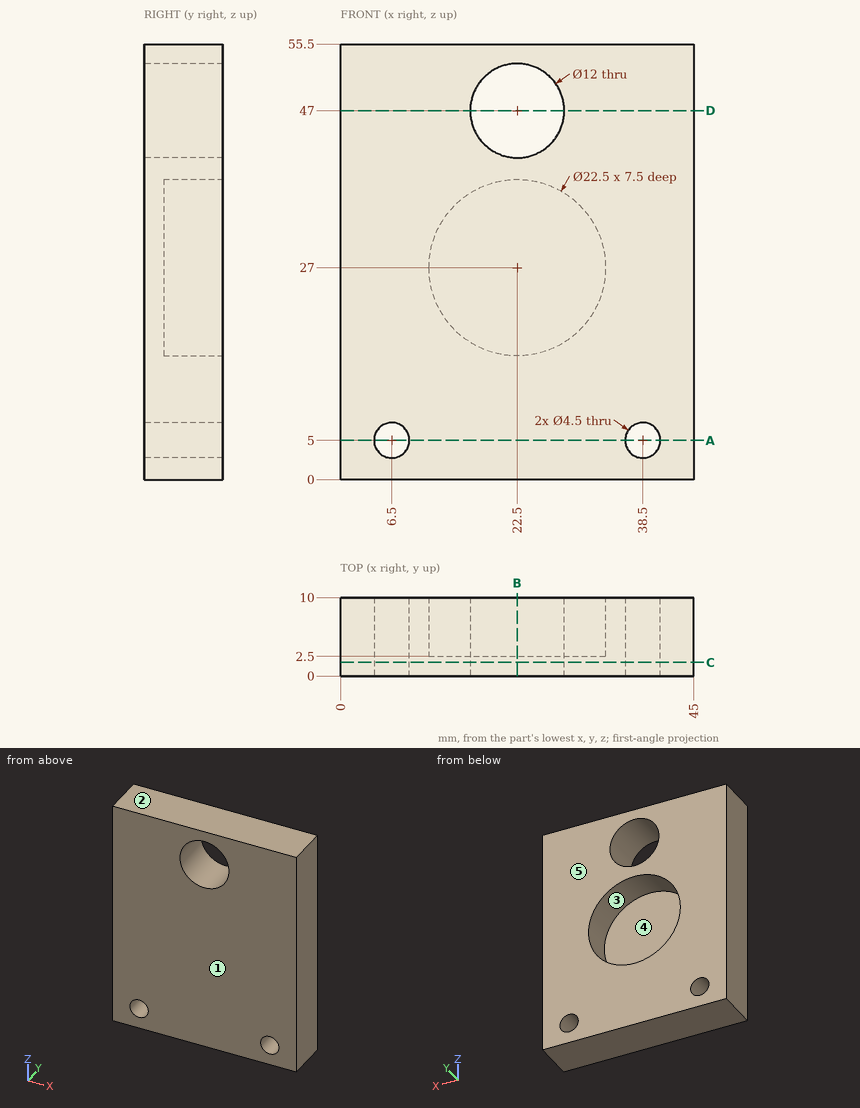
The drawing under review shows one solid part. Ordinate dimensions are in mm from its lowest x, y, z. A direction names the side the tool comes from. Round coordinates to 2 decimals unless told otherwise and drop trailing zeros. Loops run counter-clockwise (first coordinate to the right, second up) from the corner with the lowest first, then second, coordinate; pieces in that order, holes last. Notation, with made-up numbers: M 10.5,61 L 42.5,61 A12 ccw 42.5,72 Z; hole C 86.5,88.5 d11. An arc over 180 degrees is marked long. Answer as CSV lines item,"result". Start each with the question number.
Item 1: Insertion check: P1, Ø2.5, axis at x = 38.5, z = 5, coming from the -Y side; P2, Ø20, axis at x = 22.5, z = 27, coming from the +Y side. Each pin has a flat end and moves straight along its axis. Give the tip position at first contact, or say it passes through.
Item 2: Mouldability with a two-part tool opening along Z and no side actions: class the marked faces 1, 2 and 3 as released by +Z, released by -Z, zero draft, split by the parting line, or undercut.
Item 3: Consider section C-C (y = 1.75). Write out the cut boundary in (x, z), then the cut area to 3 significant figures.
Item 4: For the marked faces 4 and 5, list the 3-axis set-ups (+Z, -Z, +X, -X, +Y, -Y) from which the entire face can be reached by the end or side of a thin tool; tool diameter is ignored.
Item 5: Consider section B-B (x = 22.5). Write out the cut boundary in (y, z), then the cut area to 3 significant figures.
Item 6: Wall thickness on line 1 (Z direction, x = 22.5, y = 5.75); line 2 (Z direction, x = 6.5, y = 3.75); line 3 (Z direction, x = 17, y = 7.5): over which ranges is each line inside the solid? List them lowest first. Write a range as [from, to].
Item 7: Consider section A-A (z = 5). Write out the cut boundary in (x, y).
Item 8: Consider section D-D (z = 47). Write out the cut boundary in (x, y).
Answer:
1,P1,"passes through"
1,P2,"stops at y = 2.5"
2,face 1,"zero draft"
2,face 2,"released by +Z"
2,face 3,"undercut"
3,outline,"M 0,0 L 45,0 L 45,55.5 L 0,55.5 Z; hole C 6.5,5 d4.5; hole C 22.5,47 d12; hole C 38.5,5 d4.5"
3,area,"2,350 mm^2"
4,face 4,"+Y"
4,face 5,"+Z, -Z, +X, -X, +Y"
5,outline,"M 0,0 L 10,0 L 10,15.75 L 2.5,15.75 L 2.5,38.25 L 10,38.25 L 10,41 L 0,41 Z; M 0,53 L 10,53 L 10,55.5 L 0,55.5 Z"
5,area,"266 mm^2"
6,line 1,"z = [0, 15.75], [38.25, 41], [53, 55.5]"
6,line 2,"z = [0, 2.75], [7.25, 55.5]"
6,line 3,"z = [0, 17.19], [36.81, 44.6], [49.4, 55.5]"
7,outline,"M 0,0 L 4.25,0 L 4.25,10 L 0,10 Z; M 8.75,0 L 36.25,0 L 36.25,10 L 8.75,10 Z; M 40.75,0 L 45,0 L 45,10 L 40.75,10 Z"
8,outline,"M 0,0 L 16.5,0 L 16.5,10 L 0,10 Z; M 28.5,0 L 45,0 L 45,10 L 28.5,10 Z"
